Geometry: final body of the model. Coordinates: model frame, mm. A direction names the side the tool comes from. Coordinates: 2 decimals unless noted, no trailing zeros. Order: outer loops, then holes, each group sorted by start corner. A loop starts at its lowest first (then second) coordinate and runs counter-clockwise, first axis right, second up. Notation, with made-up numbers: M 64,59.25 L 98,59.25 A26 cw 98,83.25 Z; hole C 32.25,-36.75 d2. An arc over 180 degrees is marked long. Write item = value, one per line.
from build123d import *

# Parameters (mm, degrees)
SKETCH_1_W          = 80
SKETCH_1_H          = 50
EXTRUDE_1_DEPTH     = 40
SKETCH_2_W          = 70
SKETCH_2_H          = 40
CUT_EXTRUDE_1_DEPTH = 30
SKETCH_4_W          = 38
SKETCH_4_H          = 25
CUT_EXTRUDE_2_DEPTH = 30
SKETCH_7_W          = 80
SKETCH_7_H          = 50
SKETCH_7_W_2        = 75
SKETCH_7_H_2        = 45
CUT_EXTRUDE_3_DEPTH = 1


with BuildPart() as part:
    # 스케치1 → 보스-돌출1 (new body)
    with BuildSketch(Plane(origin=(0, 0, 0), x_dir=(1, 0, 0), z_dir=(0, 1, 0))):
        Rectangle(SKETCH_1_W, SKETCH_1_H)
    extrude(amount=EXTRUDE_1_DEPTH)

    # 스케치2 → 컷-돌출1 (cut)
    with BuildSketch(Plane.XZ):
        Rectangle(SKETCH_2_W, SKETCH_2_H)
    extrude(amount=-CUT_EXTRUDE_1_DEPTH, mode=Mode.SUBTRACT)

    # 스케치4 → 컷-돌출2 (cut)
    with BuildSketch(Plane(origin=(0, 40, 0), x_dir=(1, 0, 0), z_dir=(0, 1, 0))):
        Rectangle(SKETCH_4_W, SKETCH_4_H)
    extrude(amount=-CUT_EXTRUDE_2_DEPTH, mode=Mode.SUBTRACT)

    # 스케치7 → 컷-돌출3 (cut)
    with BuildSketch(Plane.XZ):
        Rectangle(SKETCH_7_W, SKETCH_7_H)
        Rectangle(SKETCH_7_W_2, SKETCH_7_H_2, mode=Mode.SUBTRACT)
    extrude(amount=-CUT_EXTRUDE_3_DEPTH, mode=Mode.SUBTRACT)


solid = part.part
1) Section B-B, the plane y = 15. Return loops of the section in (x, z), and give its area (3 significant figures).
Numbers:
outline = M -40,-25 L 40,-25 L 40,25 L -40,25 Z; hole M -35,-20 L 35,-20 L 35,20 L -35,20 Z
area = 1,200 mm²
2) Mould query, pull axis Z, two halves, no side actions, for faces 4 (the face through (0, 30, 14)), 5 (the face through (40, 20, 0)), 6 (the face through (-1, 20, -25)). Classes: pulls with the +Z half, pulls with the -Z half, needs draft (parallel to the pull), parting line crosses it, or undercut.
Numbers:
face_4 = undercut
face_5 = needs draft
face_6 = pulls with the -Z half
3) Line query: L1, parallel to X at y = 3, z = -6.5; L2, parallel to Z at x = -18, y = 34.5; L3, parallel to Z at x = -21.5, y = 22.5. Output: solid intervals per line, ascending.
Numbers:
L1 = -40 to -35, 35 to 40
L2 = -25 to -12.5, 12.5 to 25
L3 = -25 to -20, 20 to 25
4) Pin query (flat end, axial travel): pin 1 (1.1 mm diameter, centred on x = 4.5, y = 0.5, fed in from -Z); pin 2 (15 mm diameter, centred on x = -3.5, z = -3, fed in from -Y) (3 decimals); pin 3 (0.5 mm diameter, centred on y = 0.5, z = 8, fed in from -X). Return the tip coordinate at first contact, or that it passes through.
Numbers:
pin_1 = -25
pin_2 = through
pin_3 = -37.5
5) Section A-A, the plane x = -13.5. Return loops of the section in (y, z), and give its area (3 significant figures).
Numbers:
outline = M 0,-22.5 L 1,-22.5 L 1,-25 L 40,-25 L 40,-12.5 L 30,-12.5 L 30,-20 L 0,-20 Z; M 0,20 L 30,20 L 30,12.5 L 40,12.5 L 40,25 L 1,25 L 1,22.5 L 0,22.5 Z
area = 545 mm²
6) Section D-D, the plane x = -34. Return loops of the section in (y, z), and give its area (3 significant figures).
Numbers:
outline = M 0,-22.5 L 1,-22.5 L 1,-25 L 40,-25 L 40,25 L 1,25 L 1,22.5 L 0,22.5 L 0,20 L 30,20 L 30,-20 L 0,-20 Z
area = 795 mm²
7) Set-up query: faces 1 (the face through (-40, 20, 0)), 2 (the face through (35, 15, 0)), 3 (the face through (0, 35, -12.5)). Return all of +Z, -Z, +X, -X, +Y, -Y with unobstructed straight access to the full face (end or side cutting, diameter ignored); none if empty.
Numbers:
face_1 = +Z, -Z, -X, +Y, -Y
face_2 = -Y
face_3 = +Y, -Y
8) Section C-C, the plane z = 1. Return loops of the section in (x, y), and give its area (3 significant figures).
Numbers:
outline = M -40,1 L -37.5,1 L -37.5,0 L -35,0 L -35,30 L -19,30 L -19,40 L -40,40 Z; M 19,30 L 35,30 L 35,0 L 37.5,0 L 37.5,1 L 40,1 L 40,40 L 19,40 Z
area = 715 mm²
